from build123d import *

# Parameters (mm, degrees)
SKETCH1_W           = 76.2
SKETCH1_H           = 76.2
BOSS_EXTRUDE1_DEPTH = 12.7
SKETCH2_R           = 2.794
CUT_EXTRUDE1_DEPTH  = 56.358016583
SKETCH2_3_R         = 32.512
BOSS_EXTRUDE2_DEPTH = 5.08
FILLET1_R           = 5.08
SKETCH3_R           = 5.08
SKETCH3_R_2         = 4.1275
SKETCH3_R_3         = 1.524
CUT_EXTRUDE2_DEPTH  = 7.62
CHAMFER1_SIZE       = 1.27
CHAMFER2_SIZE       = 0.508


with BuildPart() as part:
    # Sketch1 → Boss-Extrude1 (new body)
    with BuildSketch(Plane(origin=(0, 0, 0), x_dir=(1, 0, 0), z_dir=(0, 1, 0))):
        Rectangle(SKETCH1_W, SKETCH1_H)
    extrude(amount=BOSS_EXTRUDE1_DEPTH)

    # Sketch2 → Cut-Extrude1 (cut, through all)
    with BuildSketch(Plane(origin=(0, 12.7, 0), x_dir=(1, 0, 0), z_dir=(0, 1, 0))):
        with Locations(Location((33.02, 33.02, 0), (0, 0, 270))):
            Circle(SKETCH2_R)
        with Locations(Location((33.02, -33.02, 0), (0, 0, 270))):
            Circle(SKETCH2_R)
        with Locations(Location((-33.02, -33.02, 0), (0, 0, 270))):
            Circle(SKETCH2_R)
        with Locations(Location((-33.02, 33.02, 0), (0, 0, 270))):
            Circle(SKETCH2_R)
    extrude(amount=-CUT_EXTRUDE1_DEPTH, mode=Mode.SUBTRACT)

    # Sketch2_3 → Boss-Extrude2 (add)
    with BuildSketch(Plane(origin=(0, 12.7, 0), x_dir=(1, 0, 0), z_dir=(0, 1, 0))):
        with Locations(Location((0, 0, 0), (0, 0, 90))):
            Circle(SKETCH2_3_R)
    extrude(amount=BOSS_EXTRUDE2_DEPTH)

    # Fillet1
    fillet1_edges = [part.edges().sort_by_distance(p)[0] for p in [
        (38.1, 6.35, 38.1),
        (-38.1, 6.35, 38.1),
        (-38.1, 6.35, -38.1),
        (38.1, 6.35, -38.1),
    ]]
    fillet(fillet1_edges, radius=FILLET1_R)

    # Sketch3 → Cut-Extrude2 (cut)
    # profile 1 of 8: a face of its own
    with BuildSketch(Plane(origin=(0, 17.78, 0), x_dir=(1, 0, 0), z_dir=(0, 1, 0))):
        with Locations(Location((18.306051224, 18.306051224, 0), (0, 0, 270))):
            Circle(SKETCH3_R)
        with Locations(Location((18.306051224, 18.306051224, 0), (0, 0, 270))):
            Circle(SKETCH3_R_2, mode=Mode.SUBTRACT)
    # profile 2 of 8: a face of its own
    with BuildSketch(Plane(origin=(0, 17.78, 0), x_dir=(1, 0, 0), z_dir=(0, 1, 0))):
        with Locations(Location((18.306051224, -18.306051224, 0), (0, 0, 270))):
            Circle(SKETCH3_R)
        with Locations(Location((18.306051224, -18.306051224, 0), (0, 0, 270))):
            Circle(SKETCH3_R_2, mode=Mode.SUBTRACT)
    # profile 3 of 8: a face of its own
    with BuildSketch(Plane(origin=(0, 17.78, 0), x_dir=(1, 0, 0), z_dir=(0, 1, 0))):
        with Locations(Location((-18.306051224, -18.306051224, 0), (0, 0, 270))):
            Circle(SKETCH3_R)
        with Locations(Location((-18.306051224, -18.306051224, 0), (0, 0, 270))):
            Circle(SKETCH3_R_2, mode=Mode.SUBTRACT)
    # profile 4 of 8: a face of its own
    with BuildSketch(Plane(origin=(0, 17.78, 0), x_dir=(1, 0, 0), z_dir=(0, 1, 0))):
        with Locations(Location((-18.306051224, 18.306051224, 0), (0, 0, 270))):
            Circle(SKETCH3_R)
        with Locations(Location((-18.306051224, 18.306051224, 0), (0, 0, 270))):
            Circle(SKETCH3_R_2, mode=Mode.SUBTRACT)
    # profile 5 of 8: a face of its own
    with BuildSketch(Plane(origin=(0, 17.78, 0), x_dir=(1, 0, 0), z_dir=(0, 1, 0))):
        with Locations(Location((0, 16.256, 0), (0, 0, 270))):
            Circle(SKETCH3_R_3)
    # profile 6 of 8: a face of its own
    with BuildSketch(Plane(origin=(0, 17.78, 0), x_dir=(1, 0, 0), z_dir=(0, 1, 0))):
        with Locations(Location((16.256, 0, 0), (0, 0, 270))):
            Circle(SKETCH3_R_3)
    # profile 7 of 8: a face of its own
    with BuildSketch(Plane(origin=(0, 17.78, 0), x_dir=(1, 0, 0), z_dir=(0, 1, 0))):
        with Locations(Location((0, -16.256, 0), (0, 0, 270))):
            Circle(SKETCH3_R_3)
    # profile 8 of 8: a face of its own
    with BuildSketch(Plane(origin=(0, 17.78, 0), x_dir=(1, 0, 0), z_dir=(0, 1, 0))):
        with Locations(Location((-16.256, 0, 0), (0, 0, 270))):
            Circle(SKETCH3_R_3)
    extrude(amount=-CUT_EXTRUDE2_DEPTH, mode=Mode.SUBTRACT)

    # Chamfer1
    chamfer1_edges = [part.edges().sort_by_distance(p)[0] for p in [
        (18.306051224, 17.78, 14.178551224),
        (-18.306051224, 17.78, 14.178551224),
        (-18.306051224, 17.78, -22.433551224),
        (18.306051224, 17.78, -22.433551224),
    ]]
    chamfer(chamfer1_edges, length=CHAMFER1_SIZE)

    # Chamfer2
    chamfer2_edges = [part.edges().sort_by_distance(p)[0] for p in [
        (0, 17.78, -17.78),
        (16.256, 17.78, -1.524),
        (0, 17.78, 14.732),
        (-16.256, 17.78, -1.524),
    ]]
    chamfer(chamfer2_edges, length=CHAMFER2_SIZE)


solid = part.part
Geometry check sheet. Reference: the model listing, model coordinates, mm. A direction names the side the tool comes from. Give positions to 0.01 mm unless a question says otherwise; leave off trailing zeros. Write each loop counter-clockwise with the first axis right and the second up, starting at its lowest first coordinate (ties: lowest second). Pieces come first, ordered by that corner, then holes. Notation, with made-up numbers: M 35.25,28 L 49.25,28 A18 cw 49.25,36 Z; hole C 6.25,10 d2. An arc over 180 degrees is marked long. Answer as CSV lines item,"result". Start each with the question number.
Q1. Section check C-C, the plane y = 8.5. Record the cut outline in (x, z).
Q2. Material ranges on L1, parallel to X at y = 7.25, z = 33.02; L2, parallel to X at y = 13.25, z = 0; L3, parallel to Z at x = -14, y = 15.5, recorded low to high.
Q3. Section check D-D, the plane x = -27. Record the cut outline in (y, z), then the cut area to 3 significant figures.
Q4. Release check for a two-part mould opening along X. For faces 1 (the face through (-1, 0, -1)), 2 (the face through (19.83, 14.02, -13.46)), 3 (the face through (36.572, 6.439, 36.651)) record: pulls with the +X half, pulls with the -X half, needs draft (parallel to the pull), parting line crosses it, or undercut.
Q5. Section check B-B, the plane z = 0. Record the cut outline in (x, y).
Q6. Section check A-A, the plane x = 0. Record the cut outline in (y, z), then the cut area to 3 significant figures.
Q7. Tool access check on faces 4 (the face through (0.46, 13.77, 17.71)), 5 (the face through (38.1, 6, 0)). Record the directions out of +Z, -Z, +X, -X, +Y, -Y that give a thin tool (end or side, any length) a straight path to the whole face; none if there is none.
Q8. Go/stop test with flat-tipped pins: pin 1 (4 mm diameter, centred on x = 0, z = 16.256, fed in from +Y); pin 2 (2.5 mm diameter, centred on x = 16.5, z = -0.5, fed in from +Y); pin 3 (1.5 mm diameter, centred on x = -16.5, z = 0.5, fed in from +Y); pin 4 (4.5 mm diameter, centred on x = -33.02, z = 33.02, fed in from -Y). Record where each tip stops, or that it passes through.
Geometry says:
1,outline,"M -38.1,-33.02 A5.08 ccw -33.02,-38.1 L 33.02,-38.1 A5.08 ccw 38.1,-33.02 L 38.1,33.02 A5.08 ccw 33.02,38.1 L -33.02,38.1 A5.08 ccw -38.1,33.02 Z; hole C -33.02,-33.02 d5.59; hole C -33.02,33.02 d5.59; hole C 33.02,-33.02 d5.59; hole C 33.02,33.02 d5.59"
2,L1,"-38.1 to -35.81, -30.23 to 30.23, 35.81 to 38.1"
2,L2,"-32.51 to -17.78, -14.73 to 14.73, 17.78 to 32.51"
2,L3,"-29.34 to -21, -15.61 to 15.61, 21 to 29.34"
3,outline,"M 0,-38.1 L 12.7,-38.1 L 12.7,-18.11 L 17.78,-18.11 L 17.78,18.11 L 12.7,18.11 L 12.7,38.1 L 0,38.1 Z"
3,area,"1,150 mm^2"
4,face 1,"needs draft"
4,face 2,"undercut"
4,face 3,"pulls with the +X half"
5,outline,"M -38.1,0 L 38.1,0 L 38.1,12.7 L 32.51,12.7 L 32.51,17.78 L 18.29,17.78 L 17.78,17.27 L 17.78,10.16 L 14.73,10.16 L 14.73,17.27 L 14.22,17.78 L -14.22,17.78 L -14.73,17.27 L -14.73,10.16 L -17.78,10.16 L -17.78,17.27 L -18.29,17.78 L -32.51,17.78 L -32.51,12.7 L -38.1,12.7 Z"
6,outline,"M 0,-38.1 L 12.7,-38.1 L 12.7,-32.51 L 17.78,-32.51 L 17.78,-18.29 L 17.27,-17.78 L 10.16,-17.78 L 10.16,-14.73 L 17.27,-14.73 L 17.78,-14.22 L 17.78,14.22 L 17.27,14.73 L 10.16,14.73 L 10.16,17.78 L 17.27,17.78 L 17.78,18.29 L 17.78,32.51 L 12.7,32.51 L 12.7,38.1 L 0,38.1 Z"
6,area,"1,250 mm^2"
7,face 4,"+Y"
7,face 5,"+Z, -Z, +X, +Y, -Y"
8,pin 1,"y = 17.75"
8,pin 2,"y = 17.55"
8,pin 3,"y = 10.16"
8,pin 4,"through"
